For this review, take the finished solid that the model builds, in its own axes (mm). Face numbers are marked on the shaded views. A direction names the side the tool comes from. Coordinates: 2 decimals unless noted, no trailing zeros. Write each loop counter-clockwise with the first axis right and the second up, starting at its lowest first coordinate (ties: lowest second). Pieces come first, ordered by that corner, then holes. Notation, with made-up numbers: (31.5, 19.5) -> (72.5, 19.5) arc R21 ccw to (72.5, 34.5) -> close; hole circle Ø1 at (-1, 53.25). An arc over 180 degrees is marked (long way). One line per item, written item: value. Start each with the question number.
1) Add section B-B (y = 56). State the section outline as (x, z) points.
2) For probe 1 along X at (y, z) = (71, 13); probe 2 along Z at (x, y) = (-15.5, 54); probe 3 along Y at (x, z) = (15.5, 9.5), list the stretches that pass through material, from the lowest coordinate up. Write a range as from..to.
3) Add section D-D (z = 29). State the section outline as (x, y) points.
4) For pin 1 Ø1.5 at (x, z) = (28.5, -2) entering from -Y; pin 2 Ø12.5 at (x, z) = (-18.5, -2.5) entering from +Y, all flat-tipped, find the tip position at first contact; note any pin that passes through.
5) Mouldability with a two-part tool opening along Z and no side actions: class the marked faces 3, 4 and 5 as released by +Z, released by -Z, zero draft, split by the parting line, or undercut.
6) Machinability: for the marked faces 1 and 2, which of the approach directions +Z, -Z, +X, -X, +Y, -Y give a long, thin tool a straight path to every point of the face, cutting with its end or side? Answer none if there is none.
7) Add section C-C (x = 32). State the section outline as (y, z) points, and give its area (3 significant figures).
8) Add section A-A (z = -2). State the section outline as (x, y) points, and give its area (3 significant figures).
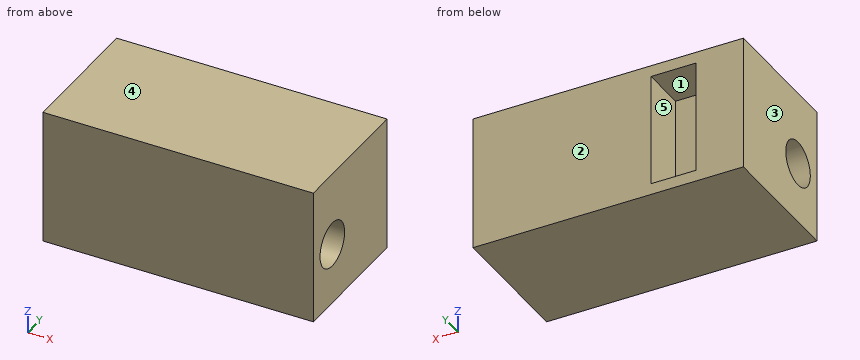
from build123d import *

# Parameters (mm, degrees)
SKETCH1_W           = 152.4
SKETCH1_H           = 76.2
BOSS_EXTRUDE1_DEPTH = 76.2
SKETCH2_R           = 12.7
CUT_EXTRUDE1_DEPTH  = 176.059416041
SKETCH3_W           = 25.4
SKETCH3_H           = 63.5
CUT_EXTRUDE2_DEPTH  = 25.4


with BuildPart() as part:
    # Sketch1 → Boss-Extrude1 (new body)
    with BuildSketch(Plane(origin=(0, 0, 0), x_dir=(1, 0, 0), z_dir=(0, 1, 0))):
        with Locations((13.452592593, -2.06962963)):
            Rectangle(SKETCH1_W, SKETCH1_H)
    extrude(amount=BOSS_EXTRUDE1_DEPTH)

    # Sketch2 → Cut-Extrude1 (cut, through all)
    with BuildSketch(Plane(origin=(89.652592593, 0, 0), x_dir=(0, 0, -1), z_dir=(1, 0, 0))):
        with Locations((1.478173536, 19.632815924)):
            Circle(SKETCH2_R)
    extrude(amount=-CUT_EXTRUDE1_DEPTH, mode=Mode.SUBTRACT)

    # Sketch3 → Cut-Extrude2 (cut)
    with BuildSketch(Plane(origin=(0, 76.2, 0), x_dir=(1, 0, 0), z_dir=(0, 1, 0))):
        with Locations((-23.407128425, -2.06962963)):
            Rectangle(SKETCH3_W, SKETCH3_H)
    extrude(amount=-CUT_EXTRUDE2_DEPTH, mode=Mode.SUBTRACT)


solid = part.part
Numbers:
1. outline: (-62.75, -36.03) -> (89.65, -36.03) -> (89.65, 40.17) -> (-62.75, 40.17) -> close; hole (-36.11, -29.68) -> (-10.71, -29.68) -> (-10.71, 33.82) -> (-36.11, 33.82) -> close
2. probe 1: -62.75..-36.11, -10.71..89.65
2. probe 2: -36.03..-29.68, 33.82..40.17
2. probe 3: 0..13.25, 26.02..76.2
3. outline: (-62.75, 0) -> (89.65, 0) -> (89.65, 76.2) -> (-10.71, 76.2) -> (-10.71, 50.8) -> (-36.11, 50.8) -> (-36.11, 76.2) -> (-62.75, 76.2) -> close
4. pin 1: y = 0
4. pin 2: y = 50.8
5. face 3: zero draft
5. face 4: released by +Z
5. face 5: undercut
6. face 1: +Y
6. face 2: +Z, -Z, +X, -X, +Y
7. outline: (0, -36.03) -> (76.2, -36.03) -> (76.2, 40.17) -> (0, 40.17) -> close; hole circle Ø25.4 at (19.63, -1.48)
7. area: 5,300 mm²
8. outline: (-62.75, 0) -> (89.65, 0) -> (89.65, 6.94) -> (-62.75, 6.94) -> close; (-62.75, 32.32) -> (89.65, 32.32) -> (89.65, 76.2) -> (-10.71, 76.2) -> (-10.71, 50.8) -> (-36.11, 50.8) -> (-36.11, 76.2) -> (-62.75, 76.2) -> close
8. area: 7,100 mm²
